from build123d import *

# Parameters (mm, degrees)
F0_R        = 11.2
F1_DEPTH    = 7
F2_T1_DEPTH = 32.0222283479
F2_T3_DEPTH = 32.0222283479
F2_T5_DEPTH = 90.1351514377
F2_T7_DEPTH = 32.0222283479
F2_T9_DEPTH = 32.0222283479
F3_T1_DEPTH = 32.0222283479
F3_T3_DEPTH = 32.0222283479
F3_T5_DEPTH = 90.1351514377
F3_T7_DEPTH = 32.0222283479
F3_T9_DEPTH = 32.0222283479


# Not quite as in the source:
# - a fillet or chamfer that OpenCascade refuses, or shapes differently, is made with other operations: its cross-section is extruded or revolved along the edge and cut away or added


with BuildPart() as f1:
    # F0 (on Top) → F1 (new body)
    with BuildSketch(Plane.XY):
        with BuildLine():
            ThreePointArc((-13.2, 0), (0, 13.2), (13.2, 0))
            Line((13.2, 0), (13.2, 38.6383682489))
            Line((13.2, 38.6383682489), (0, 52.53123492))
            Line((0, 52.53123492), (-13.2, 38.6383682489))
            Line((-13.2, 38.6383682489), (-13.2, 0))
        make_face()
        with Locations((0, 25.2957735211)):
            Circle(F0_R, mode=Mode.SUBTRACT)
        with BuildLine():
            Line((13.2, -38.6383682489), (13.2, 0))
            ThreePointArc((13.2, 0), (0, -13.2), (-13.2, 0))
            Line((-13.2, 0), (-13.2, -38.6383682489))
            Line((-13.2, -38.6383682489), (0, -52.53123492))
            Line((0, -52.53123492), (13.2, -38.6383682489))
        make_face()
        with Locations((0, -25.2957735211)):
            Circle(F0_R, mode=Mode.SUBTRACT)
        with BuildLine():
            ThreePointArc((-13.2, 0), (0, -13.2), (13.2, 0))
            ThreePointArc((13.2, 0), (0, 13.2), (-13.2, 0))
        make_face()
        Circle(F0_R, mode=Mode.SUBTRACT)
    extrude(amount=F1_DEPTH)

    # F2: chamfer of 2.5 on 6 edges, made by hand

    # F2_s2 → F2_t1 (cut)
    with BuildSketch(Plane(origin=(-30.6597100359, -32.269035129, 0), x_dir=(0, 0, 1), z_dir=(0.6887981906, 0.7249531383, 0))):
        Polygon((4.5, 36.1834195615), (7, 33.6834195615), (7, 36.1834195615), align=None)
    extrude(amount=F2_T1_DEPTH, mode=Mode.SUBTRACT)

    # F2_s4 → F2_t3 (cut)
    with BuildSketch(Plane(origin=(8.6028570917, -9.0544201944, 0), x_dir=(0, 0, 1), z_dir=(0.6887981906, -0.7249531383, 0))):
        Polygon((4.5, 36.1834195615), (7, 33.6834195615), (7, 36.1834195615), align=None)
    extrude(amount=F2_T3_DEPTH, mode=Mode.SUBTRACT)

    # F2_s6 → F2_t5 (cut)
    with BuildSketch(Plane.XZ.offset(-45.0675757189)):
        Polygon((13.2, 4.5), (10.7, 7), (13.2, 7), align=None)
        Polygon((-13.2, 4.5), (-10.7, 7), (-13.2, 7), align=None)
    extrude(amount=F2_T5_DEPTH, mode=Mode.SUBTRACT)

    # F2_s8 → F2_t7 (cut)
    with BuildSketch(Plane(origin=(30.6597100359, 32.269035129, 0), x_dir=(0, 0, 1), z_dir=(-0.6887981906, -0.7249531383, 0))):
        Polygon((4.5, 36.1834195615), (7, 33.6834195615), (7, 36.1834195615), align=None)
    extrude(amount=F2_T7_DEPTH, mode=Mode.SUBTRACT)

    # F2_s10 → F2_t9 (cut)
    with BuildSketch(Plane(origin=(-8.6028570917, 9.0544201944, 0), x_dir=(0, 0, 1), z_dir=(-0.6887981906, 0.7249531383, 0))):
        Polygon((4.5, 36.1834195615), (7, 33.6834195615), (7, 36.1834195615), align=None)
    extrude(amount=F2_T9_DEPTH, mode=Mode.SUBTRACT)

    # F3: chamfer of 2.5 on 6 edges, made by hand

    # F3_s2 → F3_t1 (cut)
    with BuildSketch(Plane(origin=(8.6028570917, -9.0544201944, 0), x_dir=(0, 0, 1), z_dir=(0.6887981906, -0.7249531383, 0))):
        Polygon((0, 33.6834195615), (2.5, 36.1834195615), (0, 36.1834195615), align=None)
    extrude(amount=F3_T1_DEPTH, mode=Mode.SUBTRACT)

    # F3_s4 → F3_t3 (cut)
    with BuildSketch(Plane(origin=(-30.6597100359, -32.269035129, 0), x_dir=(0, 0, 1), z_dir=(0.6887981906, 0.7249531383, 0))):
        Polygon((0, 33.6834195615), (2.5, 36.1834195615), (0, 36.1834195615), align=None)
    extrude(amount=F3_T3_DEPTH, mode=Mode.SUBTRACT)

    # F3_s6 → F3_t5 (cut)
    with BuildSketch(Plane.XZ.offset(-45.0675757189)):
        Polygon((10.7, 0), (13.2, 2.5), (13.2, 0), align=None)
        Polygon((-10.7, 0), (-13.2, 2.5), (-13.2, 0), align=None)
    extrude(amount=F3_T5_DEPTH, mode=Mode.SUBTRACT)

    # F3_s8 → F3_t7 (cut)
    with BuildSketch(Plane(origin=(30.6597100359, 32.269035129, 0), x_dir=(0, 0, 1), z_dir=(-0.6887981906, -0.7249531383, 0))):
        Polygon((0, 33.6834195615), (2.5, 36.1834195615), (0, 36.1834195615), align=None)
    extrude(amount=F3_T7_DEPTH, mode=Mode.SUBTRACT)

    # F3_s10 → F3_t9 (cut)
    with BuildSketch(Plane(origin=(-8.6028570917, 9.0544201944, 0), x_dir=(0, 0, 1), z_dir=(-0.6887981906, 0.7249531383, 0))):
        Polygon((2.5, 36.1834195615), (0, 33.6834195615), (0, 36.1834195615), align=None)
    extrude(amount=F3_T9_DEPTH, mode=Mode.SUBTRACT)


solid = f1.part
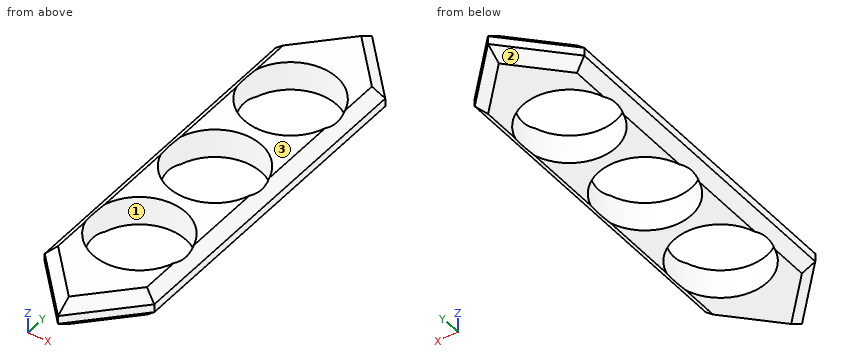
Build history of the part. All positions in model axes, mm. Face numbers are marked on the shaded views. Give positions to 0.01 mm unless a question says otherwise; leave off trailing zeros. Write each loop counter-clockwise with the first axis right and the second up, starting at its lowest first coordinate (ties: lowest second). Pieces come first, ordered by that corner, then holes. Notation, with made-up numbers: (88, 38) - (133, 38) arc R12 ccw to (133, 58) - close; hole circle Ø9 at (58.25, 56). An arc over 180 degrees is marked (long way). Use one line per item in the form item = value. Start each with the question number.
1. Band-saw the part on A-A on y = 0. Write the cut outline in (x, z).
2. Band-saw the part on B-B on x = 2. Write the cut outline in (y, z), plus the area to 3 significant figures.
3. Band-saw the part on C-C on z = 1.5. Write the cut outline in (x, y).
4. Band-saw the part on D-D on y = 21. Write the cut outline in (x, z).
5. Drop flat-ended pins along their axis: pin 1 Ø1 at (y, z) = (-37.5, 1.5) entering from -X; pin 2 Ø1.5 at (x, z) = (-2.5, 5.5) entering from +Y; pin 3 Ø2 at (x, z) = (10, 1.5) entering from -Y; pin 4 Ø10 at (x, y) = (-8.5, -24.5) entering from -Z. Give the stop position or say it passes through.
6. Probe line 1 (Y direction, x = 3.25, z = 6.75); line 2 (Y direction, x = 8.5, z = 1); line 3 (X direction, y = 0, z = 4.5). List the from-to ranges inside material, lowest first. Write a range as [from, to].
7. Two-plate mould, pull along Y, no slides. Class the marked faces 1, 2 and 3: released by +Y, released by -Y, zero draft, split by the parting line, or undercut.
Conclusion:
q1.outline = (-13.2, 2.5) - (-11.2, 0.5) - (-11.2, 6.5) - (-13.2, 4.5) - close; (11.2, 0.5) - (13.2, 2.5) - (13.2, 4.5) - (11.2, 6.5) - close
q2.outline = (-50.43, 2.5) - (-46.8, 0) - (-36.32, 0) - (-36.32, 7) - (-46.8, 7) - (-50.43, 4.5) - close; (-14.28, 0) - (-11.02, 0) - (-11.02, 7) - (-14.28, 7) - close; (11.02, 0) - (14.28, 0) - (14.28, 7) - (11.02, 7) - close; (36.32, 0) - (46.8, 0) - (50.43, 2.5) - (50.43, 4.5) - (46.8, 7) - (36.32, 7) - close
q2.area = 225 mm²
q3.outline = (-12.2, -38.24) - (0, -51.08) - (12.2, -38.24) - (12.2, 38.24) - (0, 51.08) - (-12.2, 38.24) - close; hole circle Ø22.4 at (0, -25.3); hole circle Ø22.4 at (0, 0); hole circle Ø22.4 at (0, 25.3)
q4.outline = (-13.2, 2.5) - (-10.7, 0) - (-10.34, 0) - (-10.34, 7) - (-10.7, 7) - (-13.2, 4.5) - close; (10.34, 0) - (10.7, 0) - (13.2, 2.5) - (13.2, 4.5) - (10.7, 7) - (10.34, 7) - close
q5.pin_1 = -12.7
q5.pin_2 = 49.79
q5.pin_3 = -42.35
q5.pin_4 = 0
q6.line_1 = [-45.84, -36.01], [-14.58, -10.72], [10.72, 14.58], [36.01, 45.84]
q6.line_2 = [-41.41, -32.59], [-18, -7.29], [7.29, 18], [32.59, 41.41]
q6.line_3 = [-13.2, -11.2], [11.2, 13.2]
q7.face_1 = undercut
q7.face_2 = released by +Y
q7.face_3 = zero draft
